Could you check a few things on this model? Use its own coordinates, in mm. Face numbers are marked on the shaded views. A direction names the side the tool comes from. Coordinates: 2 decimals unless noted, no trailing zeros. Return JSON: item names as keys, results as strings. Group by question number.
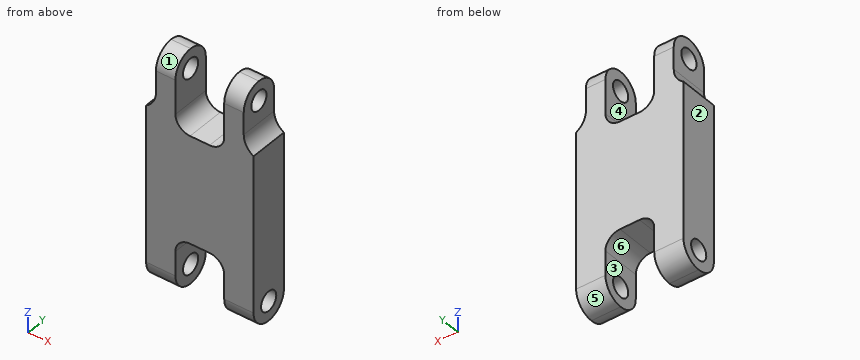
from build123d import *

# Parameters (mm, degrees)
SKETCH4_W           = 34.925
SKETCH4_H           = 12.7
BOSS_EXTRUDE2_DEPTH = 76.2
SKETCH6_W           = 15.875
SKETCH6_H           = 22.225
SKETCH6_H_2         = 19.05
CUT_EXTRUDE4_DEPTH  = 80.200182489
FILLET3_R           = 6.35
SKETCH7_R           = 3.175
CUT_EXTRUDE5_DEPTH  = 85.062584572
FILLET4_R           = 4.7625
FILLET5_R           = 4.7625
SKETCH8_W           = 3.175
SKETCH8_H           = 19.05
CUT_EXTRUDE6_DEPTH  = 80.200182489
FILLET6_R           = 6.35


# Some blends are built 0.0001 mm under size
with BuildPart() as part:
    # Sketch4 → Boss-Extrude2 (new body)
    with BuildSketch(Plane.XY):
        Rectangle(SKETCH4_W, SKETCH4_H)
    extrude(amount=BOSS_EXTRUDE2_DEPTH)

    # Sketch6 → Cut-Extrude4 (cut, through all)
    with BuildSketch(Plane(origin=(0, 6.35, 0), x_dir=(1, 0, 0), z_dir=(0, 1, 0))):
        with Locations((0, -65.0875)):
            Rectangle(SKETCH6_W, SKETCH6_H)
        with Locations((0, -9.525)):
            Rectangle(SKETCH6_W, SKETCH6_H_2)
    extrude(amount=-CUT_EXTRUDE4_DEPTH, mode=Mode.SUBTRACT)

    # Fillet3
    fillet3_edges = [part.edges().sort_by_distance(p)[0] for p in [
        (-12.7, -6.35, 0),
        (12.7, -6.35, 0),
        (-12.7, 6.35, 0),
        (12.7, 6.35, 0),
        (12.7, -6.35, 76.2),
        (12.7, 6.35, 76.2),
        (-12.7, -6.35, 76.2),
        (-12.7, 6.35, 76.2),
    ]]
    fillet(fillet3_edges, radius=FILLET3_R - 0.0001)  # a hair under: the kernel refuses the full size

    # Sketch7 → Cut-Extrude5 (cut, through all)
    with BuildSketch(Plane(origin=(17.4625, 0, 0), x_dir=(0, 0, -1), z_dir=(1, 0, 0))):
        with Locations((-6.35, 0)):
            Circle(SKETCH7_R)
        with Locations((-69.85, 0)):
            Circle(SKETCH7_R)
    extrude(amount=-CUT_EXTRUDE5_DEPTH, mode=Mode.SUBTRACT)

    # Fillet4
    fillet4_edges = [part.edges().sort_by_distance(p)[0] for p in [
        (-7.9375, 0, 19.05),
        (7.9375, 0, 19.05),
    ]]
    fillet(fillet4_edges, radius=FILLET4_R)

    # Fillet5
    fillet5_edges = [part.edges().sort_by_distance(p)[0] for p in [
        (-7.9375, 0, 53.975),
        (7.9375, 0, 53.975),
    ]]
    fillet(fillet5_edges, radius=FILLET5_R)

    # Sketch8 → Cut-Extrude6 (cut, through all)
    with BuildSketch(Plane(origin=(0, 6.35, 0), x_dir=(1, 0, 0), z_dir=(0, 1, 0))):
        with Locations((15.875, -66.675)):
            Rectangle(SKETCH8_W, SKETCH8_H)
        with Locations((-15.875, -66.675)):
            Rectangle(SKETCH8_W, SKETCH8_H)
    extrude(amount=-CUT_EXTRUDE6_DEPTH, mode=Mode.SUBTRACT)

    # Fillet6
    # the kernel refuses this fillet: 6.35 mm, written as the material it adds along each edge
    with BuildSketch(Plane(origin=(-14.2875, 6.35, 57.15), x_dir=(0, 0, 1), z_dir=(0, -1, 0))) as fillet6_piece_1:
        with BuildLine():
            CenterArc((5.499261314, 6.35), FILLET6_R, 210, 60)
            Line((0, 3.175), (-0.109985226, 3.1115))
            ThreePointArc((-0.109985226, 3.1115), (-0.127, 1.5875), (-0.127, 0))
            Line((-0.127, 0), (0, -0.127))
            Line((0, -0.127), (5.499261314, -0.127))
            Line((5.499261314, -0.127), (5.499261314, 0))
        make_face()
    extrude(amount=12.7)
    with BuildSketch(Plane(origin=(14.2875, 6.35, 57.15), x_dir=(1, 0, 0), z_dir=(0, -1, 0))) as fillet6_piece_2:
        with BuildLine():
            CenterArc((6.35, 5.499261314), FILLET6_R, 180, 60)
            Line((0, 5.499261314), (-0.127, 5.499261314))
            Line((-0.127, 5.499261314), (-0.127, 0))
            Line((-0.127, 0), (0, -0.127))
            ThreePointArc((0, -0.127), (1.5875, -0.127), (3.1115, -0.109985226))
            Line((3.1115, -0.109985226), (3.175, 0))
        make_face()
    extrude(amount=12.7)


solid = part.part
Q1. On a 3-axis mill with a long thin cutter (end or side, diameter ignored), from which of +Z, -Z, +X, -X, +Y, -Y can I reach the whole of each face in a straight line? I mean the marked faces 4, 5 and 6. Say none if no direction works.
Q2. We'd pull the mould along X, two halves only. Please class the marked faces 1, 2 and 3: pulls with the +X half, pulls with the -X half, needs draft (parallel to the pull), parting line crosses it, or undercut.
Q3. I'm going to push flat-ended pins straight in: pin 1 Ø5 at (y, z) = (0, 69.85) entering from -X; pin 2 Ø6 at (y, z) = (4.5, 63) entering from -X; pin 3 Ø1.5 at (x, y) = (-10.5, -4.5) entering from -Z; pin 4 Ø6.5 at (y, z) = (-3, 70) entering from -X. Where does each tip first touch, or does it pass through?
Q4. I need wall thicknesses on line 1 along Z through (x, y) = (-9, -0.25); line 2 along X through (y, z) = (-4, 63); line 3 along Y through (x, z) = (9.5, 69.85) (3 decimals). Which ranges of each line are inside material? Lowest first, please. Write a range as from..to.
Q5. I want a section at A-A on x = 9.5. State how many separate pieces and enclosed holes the cut face has, and give its area (3 significant figures).
Response values:
{
 "1": {"face 4": "+Z, +Y, -Y", "face 5": "-Z, +X, -X, +Y", "face 6": "-Z, +Y, -Y"},
 "2": {"face 1": "needs draft", "face 2": "pulls with the -X half", "face 3": "undercut"},
 "3": {"pin 1": "passes through", "pin 2": "stops at x = -14.87", "pin 3": "stops at z = 1.23", "pin 4": "stops at x = -14.29"},
 "4": {"line 1": "z = 0..3.18, 9.52..66.68, 73.02..76.2", "line 2": "x = -14.29..-7.94, 7.94..14.29", "line 3": "y = -6.35..-3.175, 3.175..6.35"},
 "5": {"separate pieces": "1", "enclosed holes": "2", "area": "870 mm²"}
}
